Read the model definition and answer for the solid it produces. Units are mm, in the model's axes. Face numbers are marked on the shaded views. Give positions to 0.01 mm unless a question says otherwise; leave off trailing zeros. Loops run counter-clockwise (first coordinate to the right, second up) from the corner with the lowest first, then second, coordinate; pieces in that order, holes last.
(1) Find section C-C, the plane x = -2.5. Write down the section's boundary in (y, z).
(2) Each of these flat-tipped pins is pushed along its axis until it touches: P1, Ø5, axis at x = -6, y = 6.5, coming from the +Z side; P2, Ø3.5, axis at x = 7.8, z = 5.8, coming from the -Y side; P3, Ø6, axis at x = 2.5, y = 9, coming from the -Z side; P4, Ø1.5, axis at x = 1.5, z = 5, coming from the +Y side. Where does it stop, or does it pass through?
(3) Determine the mould class of the marked faces 1, 2 and 3 for opening direction Z: pulls with the +Z half, pulls with the -Z half, needs draft (parallel to the pull), parting line crosses it, or undercut.
(4) Find section A-A, the plane x = -8.3. Write down the section's boundary in (y, z), then the cut area to 3 significant figures.
(5) Find section B-B, the plane z = -5.75. Write down the section's boundary in (x, y).
(6) Find section D-D, the plane x = 7.8. State how many separate pieces and enclosed holes the cut face has, then the cut area to 3 significant figures.
(7) Straight lines are drawn through the part: probe 1 along Z at (x, y) = (6.75, 1); probe 2 along Z at (x, y) = (-8.25, 1.5); probe 3 along Y at (x, z) = (-2.5, -7.25). For each, find the intervals that lie inside material, in ascending order.
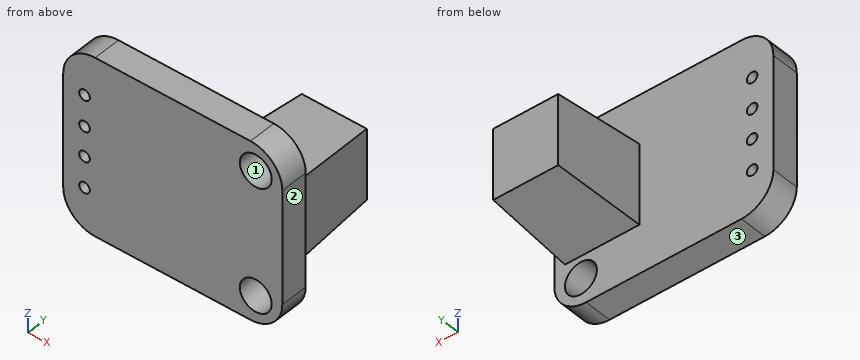
```python
from build123d import *

# Parameters (mm, degrees)
SKETCH1_W           = 20.6
SKETCH1_H           = 16.6
BOSS_EXTRUDE1_DEPTH = 2.6
FILLET1_R           = 3
SKETCH2_R           = 1.5
CUT_EXTRUDE1_DEPTH  = 2.6
SKETCH3_W           = 7
SKETCH3_H           = 7.5
BOSS_EXTRUDE2_DEPTH = 8.5
BOSS_EXTRUDE2_TAPER = 3
SKETCH4_R           = 0.5
CUT_EXTRUDE2_DEPTH  = 8.5


with BuildPart() as part:
    # Sketch1 → Boss-Extrude1 (new body)
    with BuildSketch(Plane(origin=(0, 0, 0), x_dir=(1, 0, 0), z_dir=(0, 1, 0))):
        Rectangle(SKETCH1_W, SKETCH1_H)
    extrude(amount=BOSS_EXTRUDE1_DEPTH)

    # Fillet1
    fillet1_edges = [part.edges().sort_by_distance(p)[0] for p in [
        (10.3, 1.3, 8.3),
        (-10.3, 1.3, 8.3),
        (-10.3, 1.3, -8.3),
        (10.3, 1.3, -8.3),
    ]]
    fillet(fillet1_edges, radius=FILLET1_R)

    # Sketch2 → Cut-Extrude1 (cut)
    with BuildSketch(Plane(origin=(0, 2.6, 0), x_dir=(1, 0, 0), z_dir=(0, 1, 0))):
        with Locations(Location((7.8, 5.8, 0), (0, 0, 270))):
            Circle(SKETCH2_R)
        with Locations(Location((7.8, -5.8, 0), (0, 0, 270))):
            Circle(SKETCH2_R)
    extrude(amount=-CUT_EXTRUDE1_DEPTH, mode=Mode.SUBTRACT)

    # Sketch3 → Boss-Extrude2 (add)
    with BuildSketch(Plane(origin=(0, 2.6, 0), x_dir=(1, 0, 0), z_dir=(0, 1, 0))):
        with Locations((5.8, 0)):
            Rectangle(SKETCH3_W, SKETCH3_H)
    extrude(amount=BOSS_EXTRUDE2_DEPTH, taper=BOSS_EXTRUDE2_TAPER)

    # Sketch4 → Cut-Extrude2 (cut)
    with BuildSketch(Plane(origin=(0, 2.6, 0), x_dir=(1, 0, 0), z_dir=(0, 1, 0))):
        with Locations(Location((-8.3, 4.3, 0), (0, 0, 270))):
            Circle(SKETCH4_R)
        with Locations(Location((-8.3, -4.3, 0), (0, 0, 270))):
            Circle(SKETCH4_R)
        with Locations(Location((-8.3, -1.4, 0), (0, 0, 270))):
            Circle(SKETCH4_R)
        with Locations(Location((-8.3, 1.4, 0), (0, 0, 270))):
            Circle(SKETCH4_R)
    extrude(amount=-CUT_EXTRUDE2_DEPTH, mode=Mode.SUBTRACT)


solid = part.part
```
Entries:
1. outline: (0, -8.3) - (2.6, -8.3) - (2.6, 8.3) - (0, 8.3) - close
2. P1: passes through
2. P2: stops at y = 0
2. P3: stops at z = -3.57
2. P4: stops at y = 2.6
3. face 1: undercut
3. face 2: needs draft
3. face 3: pulls with the -Z half
4. outline: (0, -8.13) - (2.6, -8.13) - (2.6, -4.8) - (0, -4.8) - close; (0, -3.8) - (2.6, -3.8) - (2.6, -1.9) - (0, -1.9) - close; (0, -0.9) - (2.6, -0.9) - (2.6, 0.9) - (0, 0.9) - close; (0, 1.9) - (2.6, 1.9) - (2.6, 3.8) - (0, 3.8) - close; (0, 4.8) - (2.6, 4.8) - (2.6, 8.13) - (0, 8.13) - close
4. area: 31.9 mm2
5. outline: (-10.27, 0) - (6.3, 0) - (6.3, 2.6) - (-10.27, 2.6) - close; (9.3, 0) - (10.27, 0) - (10.27, 2.6) - (9.3, 2.6) - close
6. separate pieces: 3
6. enclosed holes: 0
6. area: 87.3 mm2
7. probe 1: z = -8.3 to -6.87, -4.73 to 4.73, 6.87 to 8.3
7. probe 2: z = -8.15 to -4.8, -3.8 to -1.9, -0.9 to 0.9, 1.9 to 3.8, 4.8 to 8.15
7. probe 3: y = 0 to 2.6
